Source: CAD feature listing. Evaluate the final solid. Frame: model axes, mm. Face numbers are marked on the shaded views. A direction names the side the tool comes from. Give positions to 0.01 mm unless a question says otherwise; leave off trailing zeros. Write each loop counter-clockwise with the first axis right and the second up, starting at its lowest first coordinate (ties: lowest second). Pieces come first, ordered by that corner, then holes. Notation, with made-up numbers: (47.5, 29.5) -> (103.5, 29.5) arc R32 ccw to (103.5, 61.5) -> close; hole circle Ø9 at (4.25, -1.75). An arc over 180 degrees is marked (long way). Write item = value, one per line.
from build123d import *

# Parameters (mm, degrees)
F0_R     = 50.8
F1_DEPTH = 25.4
F4_DEPTH = 4.1275
F5_R     = 4.6609
F6_DEPTH = 25.401
F7_R     = 6.35
F9_DEPTH = 25.4


with BuildPart() as f1:
    # F0 (on Front) → F1 (new body)
    with BuildSketch(Plane.XZ):
        Circle(F0_R)
    extrude(amount=F1_DEPTH)

    # F3 (on face) → F4 (cut, symmetric)
    with BuildSketch(Plane.XZ.offset(25.4)):
        Polygon((4.0005, 6.9290692557), (-4.0005, 6.9290692557), (-8.001, 0), (-4.0005, -6.9290692557), (4.0005, -6.9290692557), (8.001, 0), align=None)
    extrude(amount=F4_DEPTH, both=True, mode=Mode.SUBTRACT)

    # F5 (on face) → F6 (cut, through all)
    with BuildSketch(Plane.XZ.offset(25.4)):
        Circle(F5_R)
    extrude(amount=-F6_DEPTH, mode=Mode.SUBTRACT)

    # F7
    f7_edges = [f1.edges().sort_by_distance(p)[0] for p in [
        (-50.8, -25.4, 0),
        (-50.8, 0, 0),
    ]]
    fillet(f7_edges, radius=F7_R)

    # F8 (on face) → F9 (cut, through all)
    with BuildSketch(Plane.XZ.offset(25.4)):
        with BuildLine():
            Line((4.0474563271, 44.494312185), (4.0474563271, 12.0321052626))
            ThreePointArc((4.0474563271, 12.0321052626), (10.3085981834, 7.4085263895), (12.6946232622, 0))
            ThreePointArc((12.6946232622, 0), (12.6317710989, -1.2616729662), (12.443836982, -2.5108526313))
            Line((12.443836982, -2.5108526313), (40.5569328397, -18.7419560925))
            ThreePointArc((40.5569328397, -18.7419560925), (43.6355891953, -9.594846279), (44.6780227801, 0))
            ThreePointArc((44.6780227801, 0), (32.9921056127, 30.1271752206), (4.0474563271, 44.494312185))
        make_face()
        with BuildLine():
            ThreePointArc((-12.443836982, -2.5108526313), (-10.9938662366, 6.3473116311), (-4.0474563271, 12.0321052626))
            Line((-4.0474563271, 12.0321052626), (-4.0474563271, 44.494312185))
            ThreePointArc((-4.0474563271, 44.494312185), (-38.6923027184, 22.33901139), (-40.5569328397, -18.7419560925))
            Line((-40.5569328397, -18.7419560925), (-12.443836982, -2.5108526313))
        make_face()
        with BuildLine():
            Line((36.5094765126, -25.7523560925), (8.3963806548, -9.5212526313))
            ThreePointArc((8.3963806548, -9.5212526313), (0, -12.6946232622), (-8.3963806548, -9.5212526313))
            Line((-8.3963806548, -9.5212526313), (-36.5094765126, -25.7523560925))
            ThreePointArc((-36.5094765126, -25.7523560925), (0, -44.6780227801), (36.5094765126, -25.7523560925))
        make_face()
    extrude(amount=-F9_DEPTH, mode=Mode.SUBTRACT)


solid = f1.part
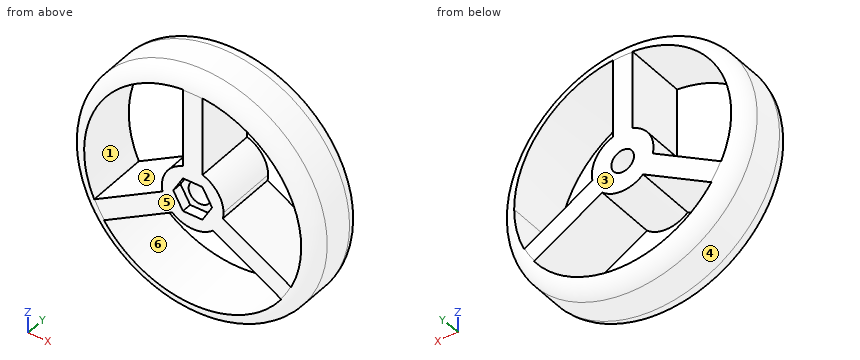
1) Cut plane A-A (y = -16.5). Return the cut outline in (x, z).
Computed:
outline = circle Ø101.6 at (0, 0); hole (-40.56, -18.74) -> (-12.44, -2.51) arc R12.69 cw to (-4.05, 12.03) -> (-4.05, 44.49) arc R44.68 ccw to start; hole (-36.51, -25.75) arc R44.68 ccw to (36.51, -25.75) -> (8.4, -9.52) arc R12.69 cw to (-8.4, -9.52) -> close; hole circle Ø9.32 at (0, 0); hole (4.05, 12.03) arc R12.69 cw to (12.44, -2.51) -> (40.56, -18.74) arc R44.68 ccw to (4.05, 44.49) -> close
2) Cut plane C-C (z = 39). State how many separate pieces and enclosed holes the cut face has, then the cut area to 3 significant figures.
Computed:
separate_pieces = 3
enclosed_holes = 0
area = 695 mm²
3) Draft query along X for the marked faces 1, 2, 3 and 4. Return one class per face: pulls with the +X half, pulls with the -X half, needs draft (parallel to the pull), parting line crosses it, or undercut.
Computed:
face_1 = undercut
face_2 = undercut
face_3 = needs draft
face_4 = parting line crosses it
4) Access query for the marked faces 5 and 6. Directions: +Z, -Z, +X, -X, +Y, -Y. A direction counts if a zero-diameter tool reaches every point of the face in a straight line with its end or side. Return the directions, or none.
Computed:
face_5 = +Z, -Z, +X, -X, -Y
face_6 = +Y, -Y
5) Material intervals for L1, parallel to Z at x = 0, y = -9.25; L2, parallel to Z at x = -5.5, y = -3.75; L3, parallel to X at y = -24, z = 36, sorted ascending.
Computed:
L1 = -50.8 to -44.68, -12.69 to -4.66, 4.66 to 50.8
L2 = -49.94 to -44.34, -11.44 to 11.44, 44.34 to 49.94
L3 = -32.39 to -26.46, -4.05 to 4.05, 26.46 to 32.39
6) Cut plane D-D (y = -2.75). Return the cut outline in (x, z), then the cut area to 3 significant figures.
Computed:
outline = circle Ø99.36 at (0, 0); hole (-40.56, -18.74) -> (-12.44, -2.51) arc R12.69 cw to (-4.05, 12.03) -> (-4.05, 44.49) arc R44.68 ccw to start; hole (-36.51, -25.75) arc R44.68 ccw to (36.51, -25.75) -> (8.4, -9.52) arc R12.69 cw to (-8.4, -9.52) -> close; hole circle Ø9.32 at (0, 0); hole (4.05, 12.03) arc R12.69 cw to (12.44, -2.51) -> (40.56, -18.74) arc R44.68 ccw to (4.05, 44.49) -> close
area = 2,700 mm²
7) Cut plane B-B (x = 0). Return the cut outline in (y, z), then the cut area to 3 significant figures.
Computed:
outline = (-25.4, -44.68) arc R6.35 ccw to (-19.05, -50.8) -> (-6.35, -50.8) arc R6.35 ccw to (0, -44.68) -> close; (-25.4, -12.69) -> (0, -12.69) -> (0, -4.66) -> (-21.27, -4.66) -> (-21.27, -6.93) -> (-25.4, -6.93) -> close; (-25.4, 6.93) -> (-21.27, 6.93) -> (-21.27, 4.66) -> (0, 4.66) -> (0, 44.45) arc R6.35 ccw to (-6.35, 50.8) -> (-19.05, 50.8) arc R6.35 ccw to (-25.4, 44.45) -> close
area = 1,480 mm²
8) Contact query for flat-ended pins moving along their axis: pin 1 (4 mm diameter, centred on x = -11.5, y = -12, fed in from +Z); pin 2 (6 mm diameter, centred on y = -17.5, z = 4.5, fed in from +X); pin 3 (8 mm diameter, centred on x = 1, y = -14.5, fed in from -Z); pin 4 (5.5 mm diameter, centred on x = 0, z = 0, fed in from -Y). Output: stop coordinate, or through.
Computed:
pin_1 = 49.9
pin_2 = 50.78
pin_3 = -50.8
pin_4 = through
